The model under review builds one solid part; all positions refer to its coordinate system, in mm. Face numbers are marked on the shaded views. A direction names the side the tool comes from. Coordinates: 2 decimals unless noted, no trailing zeros. Write each loop counter-clockwise with the first axis right and the second up, starting at its lowest first coordinate (ties: lowest second). Pieces come first, ordered by that corner, then holes. Notation, with made-up numbers: (43.5, 22.5) - (95.5, 22.5) arc R17 ccw to (95.5, 47.5) - close; hole circle Ø4 at (14.25, 79.25). An arc over 180 degrees is marked (long way). Answer as CSV lines item,"result". Start each with the question number.
```python
from build123d import *

# Parameters (mm, degrees)
F0_W     = 76.2
F0_H     = 38.1
F1_DEPTH = 25.4
F2_R     = 6.35
F3_DEPTH = 25.4
F4_R     = 11.43
F5_DEPTH = 38.1
F6_W     = 15.24
F6_H     = 12.7
F8_R     = 2.54
F9_R     = 1.27


with BuildPart() as f1:
    # F0 (on Top) → F1 (new body)
    with BuildSketch(Plane.XY):
        Rectangle(F0_W, F0_H)
    extrude(amount=F1_DEPTH)

    # F2 (on Top) → F3 (cut)
    with BuildSketch(Plane.XY):
        with Locations((-27.94, 8.89)):
            Circle(F2_R)
        with Locations((27.94, 8.89)):
            Circle(F2_R)
        with Locations((-27.94, -8.89)):
            Circle(F2_R)
        with Locations((27.94, -8.89)):
            Circle(F2_R)
    extrude(amount=F3_DEPTH, mode=Mode.SUBTRACT)

    # F4 (on face) → F5 (join)
    with BuildSketch(Plane.XY.offset(25.4)):
        Circle(F4_R)
    extrude(amount=F5_DEPTH)

    # F6 (on Front) → F7 (revolve, cut)
    with BuildSketch(Plane.XZ):
        with Locations((-16.0404087242, 42.0565381646)):
            Rectangle(F6_W, F6_H)
    revolve(axis=Axis((0, 0, 25.4), (0, 0, -1)), mode=Mode.SUBTRACT)

    # F8
    f8_edges = [f1.edges().sort_by_distance(p)[0] for p in [
        (-38.1, 0, 25.4),
        (0, -19.05, 25.4),
        (38.1, 0, 25.4),
        (0, 19.05, 25.4),
    ]]
    fillet(f8_edges, radius=F8_R)

    # F9
    f9_edges = [f1.edges().sort_by_distance(p)[0] for p in [
        (-11.43, 0, 63.5),
        (-11.43, 0, 35.706538),
        (-11.43, 0, 48.406538),
        (-11.43, 0, 25.4),
    ]]
    fillet(f9_edges, radius=F9_R)


solid = f1.part
```
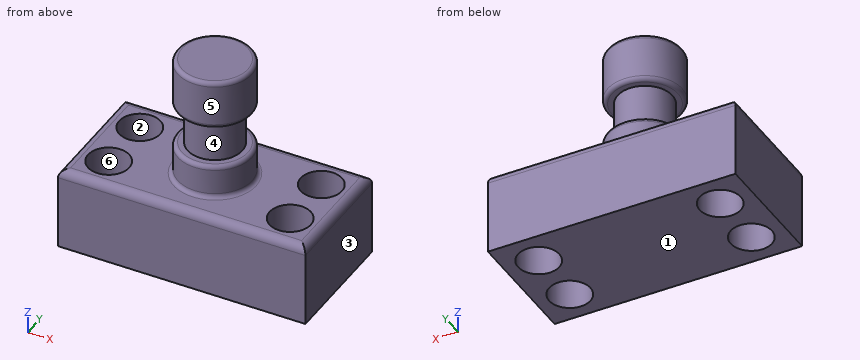
(1) For the marked faces 4, 5 and 6, list the 3-axis set-ups (+Z, -Z, +X, -X, +Y, -Y) from which the entire face can be reached by the end or side of a thin tool; tool diameter is ignored.
(2) Add section D-D on x = 0. Give the boundary of the cut face in (y, z), then the cut area to 3 significant figures.
(3) Add section B-B on z = 20. Give the boundary of the cut face in (x, y), then the cut area to 3 significant figures.
(4) For pin 1 (1 mm diameter, centred on x = 10.5, z = 56.5, fed in from +Y); pin 2 (3 mm diameter, centred on y = 0.5, z = 39.5, fed in from -X); pin 3 (20.5 mm diameter, centred on x = -27.94, y = -8.89, fed in from +Z), all flat-tipped, find the tip position at first contact; note any pin that passes through.
(5) Add section A-A on x = -27.94. Give the boundary of the cut face in (y, z), then the cut area to 3 significant figures.
(6) Add section C-C on y = 0. Give the boundary of the cut face in (x, z).
(7) Wall thickness on line 1 (Z direction, x = -2, y = 9.5); line 2 (Y direction, x = 27, z = 5); line 3 (Y direction, x = -27.94, z = 12.75): over which ranges is each line inside the solid? List them lowest first.
(8) The part is to be moulded in two halves that separate along X. For the marked faces 1, 2 and 3, say which applies: released by +X, released by -X, zero draft, split by the parting line, or undercut.
Reported:
1,face 4,"none"
1,face 5,"+Z"
1,face 6,"+Z, -Z"
2,outline,"(-19.05, 0) - (19.05, 0) - (19.05, 22.86) arc R2.54 ccw to (16.51, 25.4) - (12.7, 25.4) arc R1.27 cw to (11.43, 26.67) - (11.43, 34.44) arc R1.27 ccw to (10.16, 35.71) - (8.42, 35.71) - (8.42, 48.41) - (10.16, 48.41) arc R1.27 ccw to (11.43, 49.68) - (11.43, 62.23) arc R1.27 ccw to (10.16, 63.5) - (-10.16, 63.5) arc R1.27 ccw to (-11.43, 62.23) - (-11.43, 49.68) arc R1.27 ccw to (-10.16, 48.41) - (-8.42, 48.41) - (-8.42, 35.71) - (-10.16, 35.71) arc R1.27 ccw to (-11.43, 34.44) - (-11.43, 26.67) arc R1.27 cw to (-12.7, 25.4) - (-16.51, 25.4) arc R2.54 ccw to (-19.05, 22.86) - close"
2,area,"1,760 mm²"
3,outline,"(-38.1, -19.05) - (38.1, -19.05) - (38.1, 19.05) - (-38.1, 19.05) - close; hole circle Ø12.7 at (-27.94, -8.89); hole circle Ø12.7 at (-27.94, 8.89); hole circle Ø12.7 at (27.94, -8.89); hole circle Ø12.7 at (27.94, 8.89)"
3,area,"2,400 mm²"
4,pin 1,"y = 5.54"
4,pin 2,"x = -8.42"
4,pin 3,"z = 25.4"
5,outline,"(-19.05, 0) - (-15.24, 0) - (-15.24, 25.4) - (-16.51, 25.4) arc R2.54 ccw to (-19.05, 22.86) - close; (-2.54, 0) - (2.54, 0) - (2.54, 25.4) - (-2.54, 25.4) - close; (15.24, 0) - (19.05, 0) - (19.05, 22.86) arc R2.54 ccw to (16.51, 25.4) - (15.24, 25.4) - close"
5,area,"320 mm²"
6,outline,"(-38.1, 0) - (38.1, 0) - (38.1, 22.86) arc R2.54 ccw to (35.56, 25.4) - (12.7, 25.4) arc R1.27 cw to (11.43, 26.67) - (11.43, 34.44) arc R1.27 ccw to (10.16, 35.71) - (8.42, 35.71) - (8.42, 48.41) - (10.16, 48.41) arc R1.27 ccw to (11.43, 49.68) - (11.43, 62.23) arc R1.27 ccw to (10.16, 63.5) - (-10.16, 63.5) arc R1.27 ccw to (-11.43, 62.23) - (-11.43, 49.68) arc R1.27 ccw to (-10.16, 48.41) - (-8.42, 48.41) - (-8.42, 35.71) - (-10.16, 35.71) arc R1.27 ccw to (-11.43, 34.44) - (-11.43, 26.67) arc R1.27 cw to (-12.7, 25.4) - (-35.56, 25.4) arc R2.54 ccw to (-38.1, 22.86) - close"
7,line 1,"0 to 35.71, 48.41 to 63.5"
7,line 2,"-19.05 to -15.17, -2.61 to 2.61, 15.17 to 19.05"
7,line 3,"-19.05 to -15.24, -2.54 to 2.54, 15.24 to 19.05"
8,face 1,"zero draft"
8,face 2,"undercut"
8,face 3,"released by +X"
